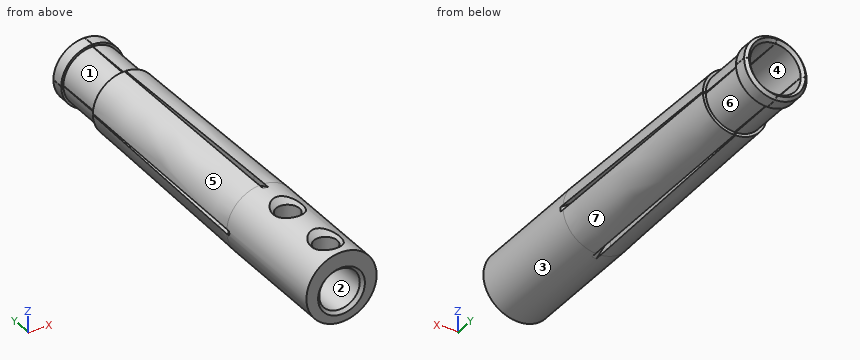
```python
from build123d import *

# Parameters (mm, degrees)
SKETCH1_W               = 4.5
SKETCH1_H               = 16
SKETCH2_R               = 3.25
CUT_EXTRUDE1_DEPTH      = 34.5
SKETCH3_R               = 2.6
CUT_EXTRUDE2_DEPTH      = 15.5
CUT_EXTRUDE3_DEPTH      = 53.964610826
CUT_EXTRUDE4_DEPTH      = 53.96461095
CUT_EXTRUDE5_DEPTH      = 0.3
CUT_EXTRUDE5_DEPTH_BACK = 0.3
CUT_EXTRUDE6_DEPTH      = 0.3
CUT_EXTRUDE6_DEPTH_BACK = 0.3
SKETCH15_R              = 4.674572256
SKETCH15_R_2            = 3.75
CUT_EXTRUDE7_DEPTH      = 6.5
CHAMFER1_SIZE           = 0.405672925
CHAMFER1_SIZE_2         = 0.4


with BuildPart() as part:
    # Sketch1 → Revolve1 (revolve)
    with BuildSketch(Plane.XY):
        Polygon((0, 16), (4.5, 16), (4, 52), (0, 52), align=None)
        with Locations((2.25, 8)):
            Rectangle(SKETCH1_W, SKETCH1_H)
    revolve(axis=Axis((0, 0, 0), (0, 1, 0)))

    # Sketch2 → Cut-Extrude1 (cut)
    with BuildSketch(Plane(origin=(0, 52, 0), x_dir=(1, 0, 0), z_dir=(0, 1, 0))):
        with Locations(Location((0, 0, 0), (0, 0, 270))):
            Circle(SKETCH2_R)
    extrude(amount=-CUT_EXTRUDE1_DEPTH, mode=Mode.SUBTRACT)

    # Sketch3 → Cut-Extrude2 (cut)
    with BuildSketch(Plane.XZ):
        with Locations(Location((0, -0.502631205, 0), (0, 0, 270))):
            Circle(SKETCH3_R)
    extrude(amount=-CUT_EXTRUDE2_DEPTH, mode=Mode.SUBTRACT)

    # Sketch5 → Cut-Extrude3 (cut, through all)
    with BuildSketch(Plane.ZY.offset(4.5)):
        Polygon((0.3, 18), (-0.3, 18), (-0.005, 52), (0.005, 52), align=None)
    extrude(amount=-CUT_EXTRUDE3_DEPTH, mode=Mode.SUBTRACT)

    # Sketch9 → Cut-Extrude4 (cut, through all)
    with BuildSketch(Plane.XY.offset(4.5)):
        Polygon((0.3, 18), (-0.3, 18), (-0.005, 52), (0.005, 52), align=None)
    extrude(amount=-CUT_EXTRUDE4_DEPTH, mode=Mode.SUBTRACT)

    # Sketch11 → Cut-Extrude5 (cut, two sides: drawn at the far end of the back side and taken through both)
    with BuildSketch(Plane.XY.offset(-CUT_EXTRUDE5_DEPTH_BACK)):
        Polygon((4.70526545, 18), (4.5, 15.5), (3.25, 18), align=None)
        Polygon((-3.25, 18), (-4.70526545, 18), (-4.5, 15.5), align=None)
    extrude(amount=CUT_EXTRUDE5_DEPTH + CUT_EXTRUDE5_DEPTH_BACK, mode=Mode.SUBTRACT)

    # Sketch14 → Cut-Extrude6 (cut, two sides: drawn at the far end of the back side and taken through both)
    with BuildSketch(Plane(origin=(0, 0, 0), x_dir=(0, 0, -1), z_dir=(1, 0, 0)).offset(-CUT_EXTRUDE6_DEPTH_BACK)):
        Polygon((4.63635838, 18), (4.5, 15.2), (3.25, 18), align=None)
        Polygon((-3.25, 18), (-4.63635838, 18), (-4.5, 15.2), align=None)
    extrude(amount=CUT_EXTRUDE6_DEPTH + CUT_EXTRUDE6_DEPTH_BACK, mode=Mode.SUBTRACT)

    # Sketch15 → Cut-Extrude7 (cut)
    with BuildSketch(Plane(origin=(0, 43.5, 0), x_dir=(1, 0, 0), z_dir=(0, 1, 0))):
        Circle(SKETCH15_R)
        Circle(SKETCH15_R_2, mode=Mode.SUBTRACT)
    extrude(amount=CUT_EXTRUDE7_DEPTH, mode=Mode.SUBTRACT)

    # CSK for M3 Oval Head Machine Screw1: read off the stored shape, not the designer's step
    # CSK for M3 Oval Head Machine Screw1 outl → CSK for M3 Oval Head Machine Screw1 (revolve, cut)
    with BuildSketch(Plane.XZ.offset(-10.8)):
        Polygon((0, 1.620808174), (1.5, 1.620808174), (1.5, 3.75), (2.250171478, 4.500171478), (0, 4.500171478), align=None)
    revolve(axis=Axis((0, 10.8, 0), (0, 0, 1)), mode=Mode.SUBTRACT)

    # CSK for M3 Oval Head Machine Screw1 2 ou → CSK for M3 Oval Head Machine Screw1 2 (revolve, cut)
    with BuildSketch(Plane.XZ.offset(-3.2)):
        Polygon((0, 1.620808174), (1.5, 1.620808174), (1.5, 3.75), (2.250171478, 4.500171478), (0, 4.500171478), align=None)
    revolve(axis=Axis((0, 3.2, 0), (0, 0, 1)), mode=Mode.SUBTRACT)

    # Chamfer1
    # the kernel refuses this chamfer: 0.405672925, 0.4 mm, written as the material it takes off along each edge
    with BuildSketch(Plane(origin=(0, 52, 0), x_dir=(-0.9664500718694985, 0, -0.2568545475233819), z_dir=(0.2568545475233819, 0, -0.9664500718694985))) as chamfer1_piece_1:
        Polygon((4 - CHAMFER1_SIZE * 0.999999998918, 0), (4 + CHAMFER1_SIZE_2 * 0.0138875494908, -CHAMFER1_SIZE_2 * 0.999903563335), (4, 0), align=None)
    revolve(axis=Axis((0, 52, 0), (0, 1, 0)), revolution_arc=119.767007275, mode=Mode.SUBTRACT)
    with BuildSketch(Plane(origin=(0, 52, 0), x_dir=(-0.2568545475233686, 0, 0.9664500718695019), z_dir=(-0.9664500718695019, 0, -0.2568545475233686))) as chamfer1_piece_2:
        Polygon((4 - CHAMFER1_SIZE * 0.999999998918, 0), (4 + CHAMFER1_SIZE_2 * 0.0138875494908, -CHAMFER1_SIZE_2 * 0.999903563335), (4, 0), align=None)
    revolve(axis=Axis((0, 52, 0), (0, 1, 0)), revolution_arc=119.767007275, mode=Mode.SUBTRACT)
    with BuildSketch(Plane(origin=(0, 52, 0), x_dir=(0.9664500718695013, 0, 0.25685454752337145), z_dir=(-0.25685454752337145, 0, 0.9664500718695013))) as chamfer1_piece_3:
        Polygon((4 - CHAMFER1_SIZE * 0.999999998918, 0), (4 + CHAMFER1_SIZE_2 * 0.0138875494908, -CHAMFER1_SIZE_2 * 0.999903563335), (4, 0), align=None)
    revolve(axis=Axis((0, 52, 0), (0, 1, 0)), revolution_arc=119.767007275, mode=Mode.SUBTRACT)
    with BuildSketch(Plane(origin=(0, 52, 0), x_dir=(0.2568545475233668, 0, -0.9664500718695025), z_dir=(0.9664500718695025, 0, 0.2568545475233668))) as chamfer1_piece_4:
        Polygon((4 - CHAMFER1_SIZE * 0.999999998918, 0), (4 + CHAMFER1_SIZE_2 * 0.0138875494908, -CHAMFER1_SIZE_2 * 0.999903563335), (4, 0), align=None)
    revolve(axis=Axis((0, 52, 0), (0, 1, 0)), revolution_arc=119.767007275, mode=Mode.SUBTRACT)
    with BuildSketch(Plane(origin=(0, 52, 0), x_dir=(-0.950764457827211, 0, -0.30991441678716625), z_dir=(0.30991441678716625, 0, -0.950764457827211))) as chamfer1_piece_5:
        Polygon((3.25, -CHAMFER1_SIZE_2), (3.25 + CHAMFER1_SIZE_2, 0), (3.25, 0), align=None)
    revolve(axis=Axis((0, 52, 0), (0, 1, 0)), revolution_arc=126.108145853, mode=Mode.SUBTRACT)
    with BuildSketch(Plane(origin=(0, 52, 0), x_dir=(-0.3099144167871693, 0, 0.9507644578272101), z_dir=(-0.9507644578272101, 0, -0.3099144167871693))) as chamfer1_piece_6:
        Polygon((3.25, -CHAMFER1_SIZE_2), (3.25 + CHAMFER1_SIZE_2, 0), (3.25, 0), align=None)
    revolve(axis=Axis((0, 52, 0), (0, 1, 0)), revolution_arc=126.108145853, mode=Mode.SUBTRACT)
    with BuildSketch(Plane(origin=(0, 52, 0), x_dir=(0.9507644578272096, 0, 0.3099144167871707), z_dir=(-0.3099144167871707, 0, 0.9507644578272096))) as chamfer1_piece_7:
        Polygon((3.25, -CHAMFER1_SIZE_2), (3.25 + CHAMFER1_SIZE_2, 0), (3.25, 0), align=None)
    revolve(axis=Axis((0, 52, 0), (0, 1, 0)), revolution_arc=126.108145853, mode=Mode.SUBTRACT)
    with BuildSketch(Plane(origin=(0, 52, 0), x_dir=(0.309914416787165, 0, -0.9507644578272114), z_dir=(0.9507644578272114, 0, 0.309914416787165))) as chamfer1_piece_8:
        Polygon((3.25, -CHAMFER1_SIZE_2), (3.25 + CHAMFER1_SIZE_2, 0), (3.25, 0), align=None)
    revolve(axis=Axis((0, 52, 0), (0, 1, 0)), revolution_arc=126.108145853, mode=Mode.SUBTRACT)
    with BuildSketch(Plane(origin=(0, 0, -0.502631205), x_dir=(0, 0, -1), z_dir=(-1, 0, 0))) as chamfer1_piece_9:
        Polygon((2.6 + CHAMFER1_SIZE_2, 0), (2.6, -CHAMFER1_SIZE_2), (2.6, 0), align=None)
    revolve(axis=Axis((0, 0, -0.502631205), (0, -1, 0)), mode=Mode.SUBTRACT)


solid = part.part
```
The model under review builds one solid part; all positions refer to its coordinate system, in mm. Face numbers are marked on the shaded views. A direction names the side the tool comes from. Round coordinates to 2 decimals unless told otherwise and drop trailing zeros. Loops run counter-clockwise (first coordinate to the right, second up) from the corner with the lowest first, then second, coordinate; pieces in that order, holes last. Notation, with made-up numbers: M -18.75,-32 L 39.25,-32 A8 cw 39.25,-20 Z; hole C 51.25,55.5 d11. An arc over 180 degrees is marked long. Answer as a JSON object with one key per item and string values.
(1) Take a section at B-B on y = 3.2. Give the boundary of the cut face in (x, z), and give its area (3 significant figures).
Resolved:
{"outline": "M -1.85,4.1 A4.5 ccw long 1.85,4.1 L 1.5,3.75 L 1.5,1.62 A2.6 cw long -1.5,1.62 L -1.5,3.75 Z", "area": "34.8 mm²"}
(2) Take a section at A-A on y = 39.5. Give the boundary of the cut face in (x, z), and give its area (3 significant figures).
Resolved:
{"outline": "M -4.17,-0.11 A4.17 ccw -0.11,-4.17 L -0.11,-3.25 A3.25 cw -3.25,-0.11 Z; M -4.17,0.11 L -3.25,0.11 A3.25 cw -0.11,3.25 L -0.11,4.17 A4.17 ccw Z; M 0.11,-4.17 A4.17 ccw 4.17,-0.11 L 3.25,-0.11 A3.25 cw 0.11,-3.25 Z; M 0.11,3.25 A3.25 cw 3.25,0.11 L 4.17,0.11 A4.17 ccw 0.11,4.17 Z", "area": "20.7 mm²"}
(3) Draft analysis for pull direction X (two halves, no side actions). For the marked faces 1, 2, 3 and 4, state which applies: released by +X, released by -X, zero draft, split by the parting line, or undercut.
Resolved:
{"face 1": "released by -X", "face 2": "undercut", "face 3": "split by the parting line", "face 4": "undercut"}
(4) Clearance check with flat-ended pins moving along their axes: P1, Ø0.6, axis at y = 16, z = -4, coming from the -X side; P2, Ø1.4, axis at x = 3.5, y = 17, coming from the -Z side; P3, Ø1, axis at y = 16, z = 3.5, coming from the +X side. State where each tip first meets the part, or that it passes through.
Resolved:
{"P1": "x = -2.56", "P2": "z = -3.51", "P3": "x = 3.35"}
(5) Take a section at C-C on x = -1. Count the separate pieces of the cut face and the enclosed holes in it, and give its area (3 significant figures).
Resolved:
{"separate pieces": "3", "enclosed holes": "0", "area": "133 mm²"}
(6) To check wall thickness, follow line 1 along Y through (x, z) = (0, 3.05); line 2 along Z through (x, y) = (0, 7); line 3 along Y through (x, z) = (-2.25, -1.75). State the ranges of each line that lie inside material, in increasing order.
Resolved:
{"line 1": "0 to 1.7, 4.7 to 9.3, 12.3 to 17.5", "line 2": "-4.5 to -3.1, 2.1 to 4.5", "line 3": "15.5 to 17.5"}
(7) Tool access review of the marked faces 5, 6 and 7: name each direction out of +Z, -Z, +X, -X, +Y, -Y from which nothing blocks a thin tool from reaching the whole face with its end or side.
Resolved:
{"face 5": "+Z, -X, +Y", "face 6": "-Z, +X", "face 7": "-Z, +X, +Y"}
(8) Take a section at D-D on y = 46.5. Give the boundary of the cut face in (x, z), and give its area (3 significant figures).
Resolved:
{"outline": "M -3.75,-0.05 A3.75 ccw -0.05,-3.75 L -0.05,-3.25 A3.25 cw -3.25,-0.05 Z; M -3.75,0.05 L -3.25,0.05 A3.25 cw -0.05,3.25 L -0.05,3.75 A3.75 ccw Z; M 0.05,-3.75 A3.75 ccw 3.75,-0.05 L 3.25,-0.05 A3.25 cw 0.05,-3.25 Z; M 0.05,3.25 A3.25 cw 3.25,0.05 L 3.75,0.05 A3.75 ccw 0.05,3.75 Z", "area": "10.8 mm²"}
